```python
from build123d import *

# Parameters (mm, degrees)
SKETCH1_W           = 46.1
SKETCH1_H           = 73.1
BOSS_EXTRUDE1_DEPTH = 1
SKETCH3_R           = 1.6
CUT_EXTRUDE1_DEPTH  = 44.222737072
SKETCH2_W           = 7.418491492
SKETCH2_H           = 57.715863808
SKETCH2_W_2         = 28.48700733
SKETCH2_H_2         = 5.638053534
BOSS_EXTRUDE2_DEPTH = 26


with BuildPart() as part:
    # Sketch1 → Boss-Extrude1 (new body)
    with BuildSketch(Plane(origin=(0, 0, 0), x_dir=(1, 0, 0), z_dir=(0, 1, 0))):
        Rectangle(SKETCH1_W, SKETCH1_H)
    extrude(amount=BOSS_EXTRUDE1_DEPTH)

    # Sketch3 → Cut-Extrude1 (cut, through all)
    with BuildSketch(Plane(origin=(0, 1, 0), x_dir=(1, 0, 0), z_dir=(0, 1, 0))):
        with Locations(Location((-18.25, 32, 0), (0, 0, 270))):
            Circle(SKETCH3_R)
        with Locations(Location((18.25, 32, 0), (0, 0, 270))):
            Circle(SKETCH3_R)
        with Locations(Location((18.25, -32, 0), (0, 0, 270))):
            Circle(SKETCH3_R)
        with Locations(Location((-18.25, -32, 0), (0, 0, 270))):
            Circle(SKETCH3_R)
    extrude(amount=-CUT_EXTRUDE1_DEPTH, mode=Mode.SUBTRACT)

    # Sketch2 → Boss-Extrude2 (add)
    with BuildSketch(Plane(origin=(0, 1, 0), x_dir=(1, 0, 0), z_dir=(0, 1, 0))):
        with Locations((-17.952749411, 0)):
            Rectangle(SKETCH2_W, SKETCH2_H)
        Rectangle(SKETCH2_W_2, SKETCH2_H)
        with Locations((0, 31.676958671)):
            Rectangle(SKETCH2_W_2, SKETCH2_H_2)
        with Locations((17.952749411, 0)):
            Rectangle(SKETCH2_W, SKETCH2_H)
        with Locations((0, -31.676958671)):
            Rectangle(SKETCH2_W_2, SKETCH2_H_2)
    extrude(amount=BOSS_EXTRUDE2_DEPTH)


solid = part.part
```
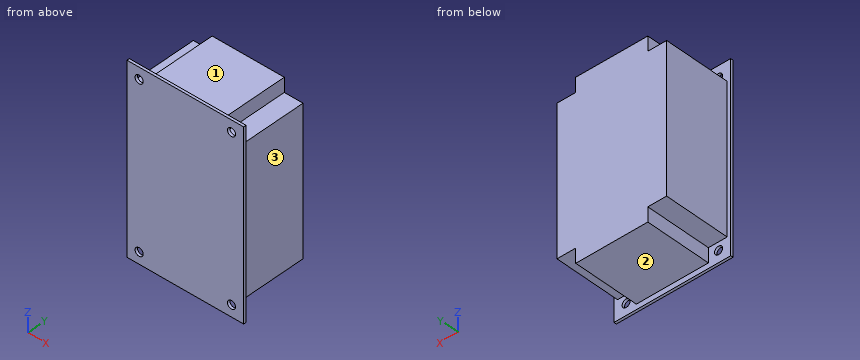
Geometry: final body of the model. Coordinates: model frame, mm. Face numbers are marked on the shaded views. A direction names the side the tool comes from. Round coordinates to 2 decimals unless told otherwise and drop trailing zeros. Order: outer loops, then holes, each group sorted by start corner. A loop starts at its lowest first (then second) coordinate and runs counter-clockwise, first axis right, second up. Notation, with made-up numbers: (33.25, 84.5) -> (56.25, 84.5) arc R19 ccw to (56.25, 114.5) -> close; hole circle Ø11 at (84, 45). An arc over 180 degrees is marked (long way). Use CSV: the item, a comma, the result in double quotes. Start each with the question number.
1) Section D-D (y = 13). Return the cut outline in (x, z).
2) Set-up query: the marked faces 1, 2 and 3. Return all of +Z, -Z, +X, -X, +Y, -Y with unobstructed straight access to the full face (end or side cutting, diameter ignored); none if empty.
3) Section B-B (z = -32). Return the cut outline in (x, y), and give its area (3 significant figures).
4) First-contact query: pin 1 Ø3 at (y, z) = (15, -32.5) entering from -X; pin 2 Ø12 at (x, y) = (-15, 22.5) entering from -Z; pin 3 Ø3 at (y, z) = (12, -32) entering from +X. Flat tips, straight axial feed; report the tip coordinate or a pass-through.
5) Section A-A (x = -18.25). Return the cut outline in (y, z), and give its area (3 significant figures).
6) Material intervals for line 1 along X through (y, z) = (0.7, -32); line 2 along X through (y, z) = (7, 24.5); line 3 along X through (y, z) = (16.5, -32), sorted ascending. Write a range as from..to.
7) Section C-C (x = 4.5). Return the cut outline in (y, z).
Returned:
1,outline,"(-21.66, -28.86) -> (-14.24, -28.86) -> (-14.24, -34.5) -> (14.24, -34.5) -> (14.24, -28.86) -> (21.66, -28.86) -> (21.66, 28.86) -> (14.24, 28.86) -> (14.24, 34.5) -> (-14.24, 34.5) -> (-14.24, 28.86) -> (-21.66, 28.86) -> close"
2,face 1,"+Z, +X, -X, +Y"
2,face 2,"-Z, +X, -X, +Y"
2,face 3,"+Z, -Z, +X, +Y"
3,outline,"(-23.05, 0) -> (-19.85, 0) -> (-19.85, 1) -> (-23.05, 1) -> close; (-16.65, 0) -> (16.65, 0) -> (16.65, 1) -> (14.24, 1) -> (14.24, 27) -> (-14.24, 27) -> (-14.24, 1) -> (-16.65, 1) -> close; (19.85, 0) -> (23.05, 0) -> (23.05, 1) -> (19.85, 1) -> close"
3,area,"780 mm²"
4,pin 1,"stops at x = -14.24"
4,pin 2,"stops at z = -34.5"
4,pin 3,"stops at x = 14.24"
5,outline,"(0, -36.55) -> (1, -36.55) -> (1, -33.6) -> (0, -33.6) -> close; (0, -30.4) -> (1, -30.4) -> (1, -28.86) -> (27, -28.86) -> (27, 28.86) -> (1, 28.86) -> (1, 30.4) -> (0, 30.4) -> close; (0, 33.6) -> (1, 33.6) -> (1, 36.55) -> (0, 36.55) -> close"
5,area,"1,570 mm²"
6,line 1,"x = -23.05..-19.85, -16.65..16.65, 19.85..23.05"
6,line 2,"x = -21.66..21.66"
6,line 3,"x = -14.24..14.24"
7,outline,"(0, -36.55) -> (1, -36.55) -> (1, -34.5) -> (27, -34.5) -> (27, 34.5) -> (1, 34.5) -> (1, 36.55) -> (0, 36.55) -> close"
